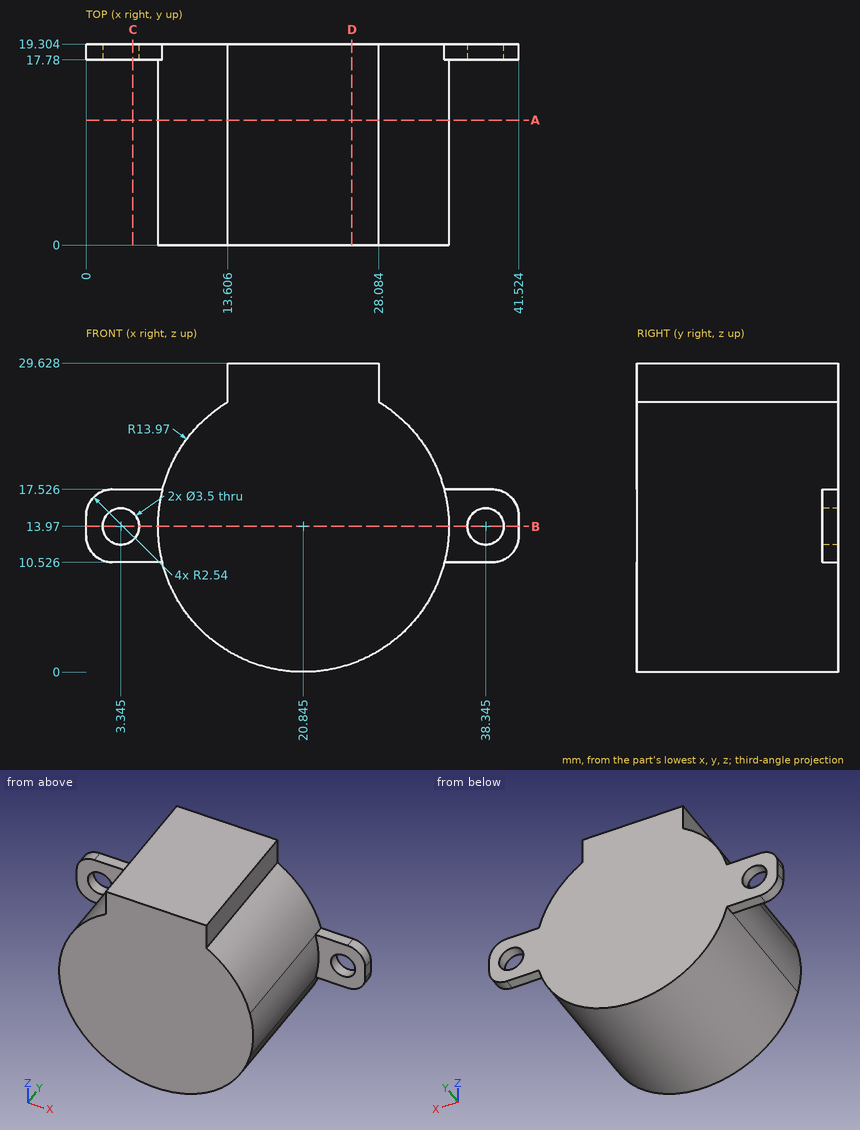
Geometry: see drawing. Coordinates: mm, zero at the bounding-box minimum. Round coordinates to 2 decimals unless told otherwise and drop trailing zeros. Loops run counter-clockwise (first coordinate to the right, second up) from the corner with the lowest first, then second, coordinate; pieces in that order, holes last. Notation, with made-up numbers: M 11.5,78 L 68.5,78 A27 cw 68.5,107 Z; hole C 24.25,-17.5 d3. An arc over 180 degrees is marked long. Use a Markdown table: item, result. Add a question column.
1. Section query B-B on z = 13.97. Return the cut outline in (x, y) (1 decimal).
2. Section query A-A on y = 12. Return the cut outline in (x, z) (1 decimal), then the cut area to 3 significant figures.
3. Contact query for flat-ended pins moving along their axis: P1, Ø4, axis at x = 12, y = 15.5, coming from the -Z side; P2, Ø6, axis at y = 10.5, z = 8.5, coming from the +X side (1 decimal); P3, Ø7.5, axis at x = 39, z = 12.5, coming from the -Y side; P4, Ø8, axis at x = 13.5, y = 11.5, coming from the +Z side. Output: stop coordinate, or through.
4. Section query D-D on x = 25.5. Return the cut outline in (y, z).
5. Section query C-C on x = 4.5. Return the cut outline in (y, z) (1 decimal).
6. Line query: line 1 (X direction, y = 18.8, z = 13.97) (1 decimal); line 2 (X direction, y = 13.25, z = 13.5); line 3 (Y direction, x = 7, z = 10.75). Output: solid intervals per line, ascending.
Reported:
| question | item | result |
|---|---|---|
| 1 | outline | M 0,17.8 L 1.6,17.8 L 1.6,19.3 L 0,19.3 Z; M 5.1,17.8 L 6.9,17.8 L 6.9,0 L 34.8,0 L 34.8,17.8 L 36.6,17.8 L 36.6,19.3 L 5.1,19.3 Z; M 40.1,17.8 L 41.5,17.8 L 41.5,19.3 L 40.1,19.3 Z |
| 2 | outline | M 13.6,25.9 A14 ccw long 28.1,25.9 L 28.1,29.6 L 13.6,29.6 Z |
| 2 | area | 647 mm² |
| 3 | P1 | stops at z = 1.79 |
| 3 | P2 | stops at x = 34.6 |
| 3 | P3 | stops at y = 17.78 |
| 3 | P4 | stops at z = 29.63 |
| 4 | outline | M 0,0.8 L 19.3,0.8 L 19.3,29.63 L 0,29.63 Z |
| 5 | outline | M 17.8,10.5 L 19.3,10.5 L 19.3,12.7 L 17.8,12.7 Z; M 17.8,15.3 L 19.3,15.3 L 19.3,17.5 L 17.8,17.5 Z |
| 6 | line 1 | x = 0 to 1.6, 5.1 to 36.6, 40.1 to 41.5 |
| 6 | line 2 | x = 6.88 to 34.81 |
| 6 | line 3 | y = 17.78 to 19.3 |
